Geometry check sheet. Reference: the model listing, model coordinates, mm. Round coordinates to 2 decimals unless told otherwise and drop trailing zeros. Write each loop counter-clockwise with the first axis right and the second up, starting at its lowest first coordinate (ties: lowest second). Pieces come first, ordered by that corner, then holes. Notation, with made-up numbers: M 85.5,66 L 126.5,66 A23 ccw 126.5,74 Z; hole C -4,-31 d11. An arc over 180 degrees is marked long. Use a Markdown table: item, result.
```python
from build123d import *

# Parameters (mm, degrees)
SKETCH1_W           = 10
SKETCH1_H           = 1
BOSS_EXTRUDE1_DEPTH = 2
FILLET1_RADIUS      = 1
FILLET1_LENGTH      = 1
FILLET2_RADIUS      = 0.5
FILLET2_LENGTH      = 2


with BuildPart() as part:
    # Sketch1 → Boss-Extrude1 (new body)
    with BuildSketch(Plane.XY):
        with Locations((0.174129353, -0.226368159)):
            Rectangle(SKETCH1_W, SKETCH1_H)
    extrude(amount=BOSS_EXTRUDE1_DEPTH)

    # Fillet1: full round fillet: the end face becomes a half cylinder, R = half its width
    fillet1_face = Plane((5.174129353, -0.226368159, 1), x_dir=(0, -1, 0), z_dir=(1, 0, 0))  # on the end face: x along it, z out of the body
    fillet1_slab = fillet1_face.offset(-FILLET1_RADIUS / 2) * Box(FILLET1_LENGTH, 2 * FILLET1_RADIUS, FILLET1_RADIUS, mode=Mode.PRIVATE)  # the body's end, R deep
    fillet1_round = Plane((4.174129353, -0.226368159, 1), x_dir=(1, 0, 0), z_dir=(0, -1, 0)) * Cylinder(FILLET1_RADIUS, FILLET1_LENGTH, mode=Mode.PRIVATE)  # its axis R under the face
    add(fillet1_slab - fillet1_round, mode=Mode.SUBTRACT)

    # Fillet2: full round fillet: the end face becomes a half cylinder, R = half its width
    fillet2_face = Plane((-4.825870647, -0.226368159, 1), x_dir=(0, 0, -1), z_dir=(-1, 0, 0))  # on the end face: x along it, z out of the body
    fillet2_slab = fillet2_face.offset(-FILLET2_RADIUS / 2) * Box(FILLET2_LENGTH, 2 * FILLET2_RADIUS, FILLET2_RADIUS, mode=Mode.PRIVATE)  # the body's end, R deep
    fillet2_round = Plane((-4.325870647, -0.226368159, 1), x_dir=(-1, 0, 0), z_dir=(0, 0, -1)) * Cylinder(FILLET2_RADIUS, FILLET2_LENGTH, mode=Mode.PRIVATE)  # its axis R under the face
    add(fillet2_slab - fillet2_round, mode=Mode.SUBTRACT)


solid = part.part
```
Item 1: Cross-section at B-B, the plane y = 0. Record the cut outline in (x, z).
Outcome:
| item | result |
|---|---|
| outline | M -4.77,0 L 4.17,0 A1 ccw 4.17,2 L -4.77,2 Z |
Item 2: Material ranges on line 1 along Z through (x, y) = (4.25, -0.5); line 2 along X through (y, z) = (-0.25, 0.5); line 3 along X through (y, z) = (-0.55, 0.9), recorded low to high. Write a range as from..to.
Outcome:
| item | result |
|---|---|
| line 1 | z = 0..2 |
| line 2 | x = -4.83..5.04 |
| line 3 | x = -4.71..5.17 |
Item 3: Cross-section at A-A, the plane z = 1.6. Record the cut outline in (x, y), and give its area (3 significant figures).
Outcome:
| item | result |
|---|---|
| outline | M -4.33,-0.73 L 4.97,-0.73 L 4.97,0.27 L -4.33,0.27 A0.5 ccw Z |
| area | 9.69 mm2 |
